Read the model definition and answer for the solid it produces. Units are mm, in the model's axes. Face numbers are marked on the shaded views. A direction names the side the tool comes from. Coordinates: 2 decimals unless noted, no trailing zeros. Write each loop counter-clockwise with the first axis right and the second up, starting at its lowest first coordinate (ties: lowest second). Pieces come first, ordered by that corner, then holes. Notation, with made-up numbers: (63.25, -32) -> (99.25, -32) arc R32 cw to (99.25, -5) -> close; hole circle Ø4 at (84.25, 70). An arc over 180 degrees is marked (long way). Write item = value, one per line. Start each with the question number.
1) Section B-B (z = 6.5) is taken. Determine the outline of the cut face in (x, y).
2) For a pull along X with two mould halves and no side action, classify the marked faces 1, 2 and 3 as released by +X, released by -X, zero draft, split by the parting line, or undercut.
3) Section D-D (x = 14) is taken. Determine the outline of the cut face in (y, z).
4) Find the intervals of material crossed by line 1 along Y through (x, z) = (0, 6.15); line 2 along Y through (x, z) = (0, 3.75); line 3 along Z through (x, y) = (-4, -18), in increasing order. Write a range as from..to.
5) Flat-ended cylindrical pins translate along their axes: pin 1 Ø4.5 at (y, z) = (-5, 4) entering from -X (3 decimals); pin 2 Ø3 at (x, z) = (-3, 2) entering from +Y; pin 3 Ø1.5 at (x, z) = (-2, 3.5) entering from -Y. Find the tip coordinate at first contact, or state that the pin passes through.
6) Section A-A (x = 0) is taken. Determine the outline of the cut face in (y, z).
7) Section C-C (y = 0) is taken. Determine the outline of the cut face in (x, z).
8) A tool of negligible diameter and unlimited length cuts with its end or side. For the marked faces 4, 5 and 6, from which of +Z, -Z, +X, -X, +Y, -Y can it reach the whole face along a straight path? Write none if from no direction.
from build123d import *

# Parameters (mm, degrees)
SKETCH_R        = 23
PAD_DEPTH       = 5
SKETCH001_W     = 13
SKETCH001_H     = 22
POCKET_DEPTH    = 4
SKETCH002_W     = 11
SKETCH002_H     = 5
POCKET001_DEPTH = 1.001
SKETCH008_R     = 20
SKETCH008_R_2   = 19
PAD005_DEPTH    = 3
SKETCH011_R     = 23
SKETCH011_R_2   = 21.3
POCKET002_DEPTH = 4


with BuildPart() as part:
    # Sketch → Pad (new body)
    with BuildSketch(Plane.XY):
        Circle(SKETCH_R)
    extrude(amount=PAD_DEPTH)

    # Sketch001 (on Face3 of Pad) → Pocket (cut)
    with BuildSketch(Plane.XY.offset(5)):
        Rectangle(SKETCH001_W, SKETCH001_H)
    extrude(amount=-POCKET_DEPTH, mode=Mode.SUBTRACT)

    # Sketch002 (on Face8 of Pocket) → Pocket001 (cut, through all)
    with BuildSketch(Plane.XY.offset(1)):
        with Locations((0, 8.5)):
            Rectangle(SKETCH002_W, SKETCH002_H)
    extrude(amount=-POCKET001_DEPTH, mode=Mode.SUBTRACT)

    # Sketch008 → Pad005 (join)
    with BuildSketch(Plane.XY.offset(5)):
        Circle(SKETCH008_R)
        Circle(SKETCH008_R_2, mode=Mode.SUBTRACT)
    extrude(amount=PAD005_DEPTH)

    # Sketch011 (on Face2 of Pad005) → Pocket002 (cut)
    with BuildSketch(Plane(origin=(0, 0, 0), x_dir=(1, 0, 0), z_dir=(0, 0, -1))):
        Circle(SKETCH011_R)
        Circle(SKETCH011_R_2, mode=Mode.SUBTRACT)
    extrude(amount=-POCKET002_DEPTH, mode=Mode.SUBTRACT)


solid = part.part
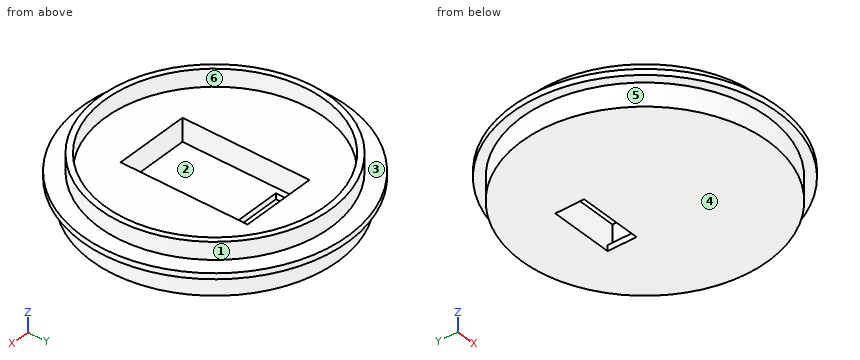
Answer key:
q1.outline = circle Ø40 at (0, 0); hole circle Ø38 at (0, 0)
q2.face_1 = split by the parting line
q2.face_2 = undercut
q2.face_3 = zero draft
q3.outline = (-18.25, 4) -> (-16.05, 4) -> (-16.05, 0) -> (16.05, 0) -> (16.05, 4) -> (18.25, 4) -> (18.25, 5) -> (14.28, 5) -> (14.28, 8) -> (12.85, 8) -> (12.85, 5) -> (-12.85, 5) -> (-12.85, 8) -> (-14.28, 8) -> (-14.28, 5) -> (-18.25, 5) -> close
q4.line_1 = -20..-19, 19..20
q4.line_2 = -21.3..-11, 11..21.3
q4.line_3 = 0..5
q5.pin_1 = -22.835
q5.pin_2 = 21.25
q5.pin_3 = -22.95
q6.outline = (-23, 4) -> (-21.3, 4) -> (-21.3, 0) -> (6, 0) -> (6, 1) -> (-11, 1) -> (-11, 5) -> (-19, 5) -> (-19, 8) -> (-20, 8) -> (-20, 5) -> (-23, 5) -> close; (11, 0) -> (21.3, 0) -> (21.3, 4) -> (23, 4) -> (23, 5) -> (20, 5) -> (20, 8) -> (19, 8) -> (19, 5) -> (11, 5) -> close
q7.outline = (-23, 4) -> (-21.3, 4) -> (-21.3, 0) -> (21.3, 0) -> (21.3, 4) -> (23, 4) -> (23, 5) -> (20, 5) -> (20, 8) -> (19, 8) -> (19, 5) -> (6.5, 5) -> (6.5, 1) -> (-6.5, 1) -> (-6.5, 5) -> (-19, 5) -> (-19, 8) -> (-20, 8) -> (-20, 5) -> (-23, 5) -> close
q8.face_4 = -Z, +X, -X, +Y, -Y
q8.face_5 = -Z
q8.face_6 = +Z
